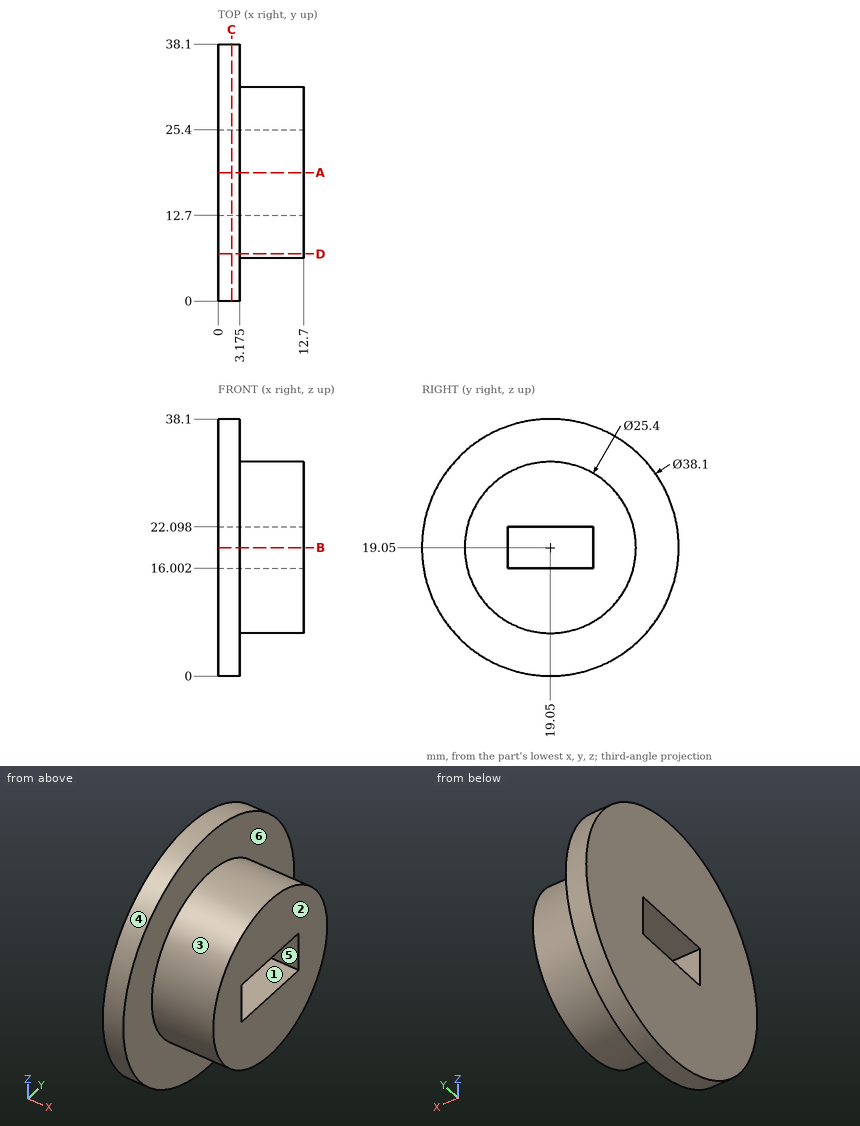
Could you check a few things on this drawing? It's one solid part, dimensions in mm from its lowest x, y, z. A direction names the side the tool comes from. Round coordinates to 2 decimals unless told otherwise and drop trailing zeros. Order: outer loops, then holes, each group sorted by start corner. A loop starts at its lowest first (then second) coordinate and runs counter-clockwise, first axis right, second up. Notation, with made-up numbers: M -16,-28.5 L 41,-28.5 A19 cw 41,-4.5 Z; hole C 70.5,31.25 d4. An arc over 180 degrees is marked long. Return JSON: item names as keys, results as strings. Group by question number.
1. If we mould it in two halves opening along Y, with no side actions, what happens to the marked faces 4, 5 and 6? For each: pulls with the +Y half, pulls with the -Y half, needs draft (parallel to the pull), parting line crosses it, or undercut.
2. If we section it at B-B on z = 19.05: List the corners of the cut face in (x, y) for me (3 decimals).
3. Please list where these lines run through material, in increasing order: probe 1 along Z at (x, y) = (7.5, 19); probe 2 along Y at (x, z) = (1, 18.5); probe 3 along Z at (x, y) = (5.5, 15).
4. If we section it at A-A on y = 19.05: List the corners of the cut face in (x, z) for me (3 decimals).
5. On a 3-axis mill with a long thin cutter (end or side, diameter ignored), from which of +Z, -Z, +X, -X, +Y, -Y can I reach the whole of each face in a straight line? I mean the marked faces 1, 2 and 3. Say none if no direction works.
6. If we section it at D-D on y = 7: List the corners of the cut face in (x, z) for me (3 decimals).
7. I'm going to push flat-ended pins straight in: pin 1 Ø5 at (x, z) = (9.5, 31.5) entering from -Y; pin 2 Ø3 at (x, z) = (9, 18.5) entering from -Y; pin 3 Ø4 at (x, z) = (11, 7.5) entering from -Y. Where does each tip first touch, or does it pass through?
8. If we section it at C-C on x = 2: List the corners of the cut face in (y, z) for me, then the cut area to 3 significant figures.
Reply:
{
 "1": {"face 4": "parting line crosses it", "face 5": "undercut", "face 6": "needs draft"},
 "2": {"outline": "M 0,0 L 3.175,0 L 3.175,6.35 L 12.7,6.35 L 12.7,12.7 L 0,12.7 Z; M 0,25.4 L 12.7,25.4 L 12.7,31.75 L 3.175,31.75 L 3.175,38.1 L 0,38.1 Z"},
 "3": {"probe 1": "6.35 to 16, 22.1 to 31.75", "probe 2": "0.01 to 12.7, 25.4 to 38.09", "probe 3": "7.01 to 16, 22.1 to 31.09"},
 "4": {"outline": "M 0,0 L 3.175,0 L 3.175,6.35 L 12.7,6.35 L 12.7,16.002 L 0,16.002 Z; M 0,22.098 L 12.7,22.098 L 12.7,31.75 L 3.175,31.75 L 3.175,38.1 L 0,38.1 Z"},
 "5": {"face 1": "+X, -X", "face 2": "+Z, -Z, +X, +Y, -Y", "face 3": "+X"},
 "6": {"outline": "M 0,4.295 L 3.175,4.295 L 3.175,15.039 L 12.7,15.039 L 12.7,23.061 L 3.175,23.061 L 3.175,33.805 L 0,33.805 Z"},
 "7": {"pin 1": "y = 11.16", "pin 2": "y = 6.35", "pin 3": "y = 10.68"},
 "8": {"outline": "C 19.05,19.05 d38.1; hole M 12.7,16 L 25.4,16 L 25.4,22.1 L 12.7,22.1 Z", "area": "1,060 mm^2"}
}
